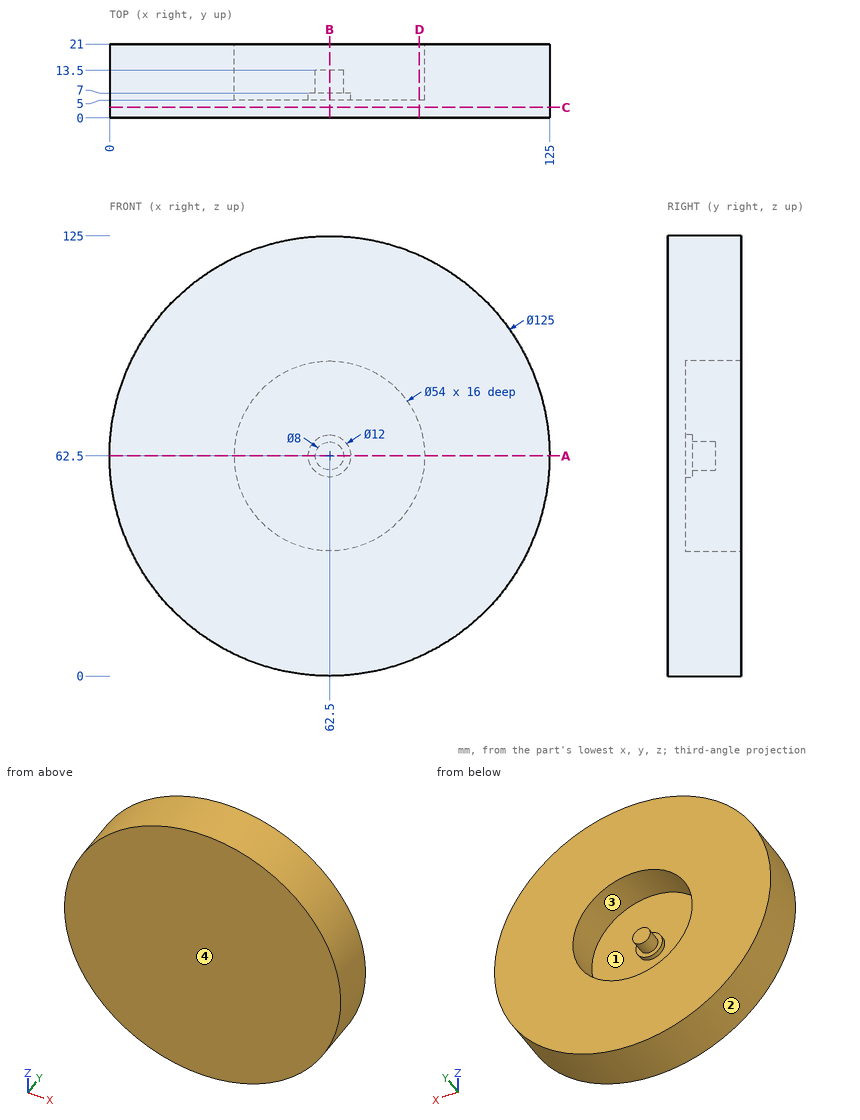
Input: dimensioned drawing with shaded views. Units: mm. Origin: part minimum x, y, z. Round coordinates to 2 decimals unless told otherwise and drop trailing zeros. Write each loop counter-clockwise with the first axis right and the second up, starting at its lowest first coordinate (ties: lowest second). Pieces come first, ordered by that corner, then holes. Notation, with made-up numbers: (28.25, 43.25) -> (62.25, 43.25) arc R16 ccw to (62.25, 70.25) -> close; hole circle Ø2 at (41.5, 35). An arc over 180 degrees is marked (long way). Use CSV: the item, a comma, the result in double quotes. Start each with the question number.
Q1. Line query: L1, parallel to X at y = 17, z = 62.5; L2, parallel to X at y = 9.5, z = 62.5; L3, parallel to Y at x = 85, z = 54.5. Output: solid intervals per line, ascending.
Q2. First-contact query: pin 1 Ø6 at (x, z) = (60.5, 63.5) entering from +Y; pin 2 Ø16 at (x, z) = (56, 73) entering from +Y; pin 3 Ø6 at (y, z) = (14.5, 34) entering from +X. Flat tips, straight axial feed; report the tip coordinate or a pass-through.
Q3. Section D-D (x = 88). Return loops of the section in (y, z), plus the area to 3 significant figures.
Q4. Section B-B (x = 62.5). Return loops of the section in (y, z).
Q5. Section A-A (z = 62.5). Return loops of the section in (x, y), plus the area to 3 significant figures.
Q6. Section C-C (y = 3). Return loops of the section in (x, z), plus the area to 3 significant figures.
Q7. Pull-direction query (Z, two-part tool) for the marked faces 1, 2, 3 and 4; classes: pulls with the +Z half, pulls with the -Z half, needs draft (parallel to the pull), parting line crosses it, or undercut.
Result sheet:
1,L1,"0 to 35.5, 89.5 to 125"
1,L2,"0 to 35.5, 58.5 to 66.5, 89.5 to 125"
1,L3,"0 to 5"
2,pin 1,"y = 13.5"
2,pin 2,"y = 7"
2,pin 3,"x = 119.56"
3,outline,"(0, 5.44) -> (21, 5.44) -> (21, 53.63) -> (5, 53.63) -> (5, 71.37) -> (21, 71.37) -> (21, 119.56) -> (0, 119.56) -> close"
3,area,"2,110 mm²"
4,outline,"(0, 0) -> (21, 0) -> (21, 35.5) -> (5, 35.5) -> (5, 56.5) -> (7, 56.5) -> (7, 58.5) -> (13.5, 58.5) -> (13.5, 66.5) -> (7, 66.5) -> (7, 68.5) -> (5, 68.5) -> (5, 89.5) -> (21, 89.5) -> (21, 125) -> (0, 125) -> close"
5,outline,"(0, 0) -> (125, 0) -> (125, 21) -> (89.5, 21) -> (89.5, 5) -> (68.5, 5) -> (68.5, 7) -> (66.5, 7) -> (66.5, 13.5) -> (58.5, 13.5) -> (58.5, 7) -> (56.5, 7) -> (56.5, 5) -> (35.5, 5) -> (35.5, 21) -> (0, 21) -> close"
5,area,"1,840 mm²"
6,outline,"circle Ø125 at (62.5, 62.5)"
6,area,"12,300 mm²"
7,face 1,"undercut"
7,face 2,"parting line crosses it"
7,face 3,"undercut"
7,face 4,"needs draft"
